from build123d import *

# Parameters (mm, degrees)
F1_DEPTH = 25.4
F2_W     = 381
F2_H     = 12.7
F4_DEPTH = 304.8
F3_W     = 203.2
F3_H     = 76.2
F5_DEPTH = 50.8


with BuildPart() as f1:
    # F0 (on Top) → F1 (new body)
    with BuildSketch(Plane.XY):
        Polygon((-208.403401, 57.177154), (-208.403401, -196.822846), (172.596599, -196.822846), (172.596599, 57.177154), (83.696599, 57.177154), (-119.503401, 57.177154), align=None)
    extrude(amount=F1_DEPTH)

    # F2 (on Top) → F4 (join)
    with BuildSketch(Plane.XY):
        with Locations((-17.903401, 63.527154)):
            Rectangle(F2_W, F2_H)
    extrude(amount=F4_DEPTH)

    # F3 (on Top) → F5 (join)
    with BuildSketch(Plane.XY):
        with Locations((-17.903401, 107.977154)):
            Rectangle(F3_W, F3_H)
    extrude(amount=F5_DEPTH)


solid = f1.part
Source: CAD feature listing. Evaluate the final solid. Frame: model axes, mm. A direction names the side the tool comes from. Give positions to 0.01 mm unless a question says otherwise; leave off trailing zeros. Order: outer loops, then holes, each group sorted by start corner. A loop starts at its lowest first (then second) coordinate and runs counter-clockwise, first axis right, second up. Notation, with made-up numbers: (37.25, 85) -> (86.25, 85) arc R17 ccw to (86.25, 108) -> close; hole circle Ø5 at (-7.5, -33.75). An arc over 180 degrees is marked (long way). Write item = value, one per line.
Q1. Pin query (flat end, axial travel): pin 1 (3 mm diameter, centred on x = -34, z = 122.5, fed in from -Y); pin 2 (3 mm diameter, centred on x = -74, z = 52.5, fed in from +Y); pin 3 (10 mm diameter, centred on x = -51.5, y = -133, fed in from +Z). Return the tip coordinate at first contact, or that it passes through.
Data:
pin_1 = 57.18
pin_2 = 69.88
pin_3 = 25.4
Q2. Cut plane C-C, the plane z = 240.5. Output: boundary loops of the cut face in (x, y), and give its area (3 significant figures).
Data:
outline = (-208.4, 57.18) -> (172.6, 57.18) -> (172.6, 69.88) -> (-208.4, 69.88) -> close
area = 4,840 mm^2
Q3. Cut plane B-B, the plane y = -137.5. Output: boundary loops of the cut face in (x, z), and give its area (3 significant figures).
Data:
outline = (-208.4, 0) -> (172.6, 0) -> (172.6, 25.4) -> (-208.4, 25.4) -> close
area = 9,680 mm^2
Q4. Cut plane D-D, the plane x = -180.5. Output: boundary loops of the cut face in (y, z).
Data:
outline = (-196.82, 0) -> (69.88, 0) -> (69.88, 304.8) -> (57.18, 304.8) -> (57.18, 25.4) -> (-196.82, 25.4) -> close
Q5. Set-up query: faces 1 (the face through (83.697, 107, 25)), 2 (the face through (-19, 109, 50.8)), 3 (the face through (-21, -68, 25.4)). Return all of +Z, -Z, +X, -X, +Y, -Y with unobstructed straight access to the full face (end or side cutting, diameter ignored); none if empty.
Data:
face_1 = +Z, -Z, +X, +Y
face_2 = +Z, +X, -X, +Y
face_3 = +Z, +X, -X, -Y
Q6. Cut plane A-A, the plane x = -79.5. Output: boundary loops of the cut face in (y, z), and give its area (3 significant figures).
Data:
outline = (-196.82, 0) -> (146.08, 0) -> (146.08, 50.8) -> (69.88, 50.8) -> (69.88, 304.8) -> (57.18, 304.8) -> (57.18, 25.4) -> (-196.82, 25.4) -> close
area = 14,200 mm^2
Q7. Material intervals for line 1 (Z direction, x = -68.5, y = -17); line 2 (Y direction, x = 141, z = 242); line 3 (Y direction, x = 124.5, z = 17.5), sorted ascending. Write a range as from..to.
Data:
line_1 = 0..25.4
line_2 = 57.18..69.88
line_3 = -196.82..69.88
